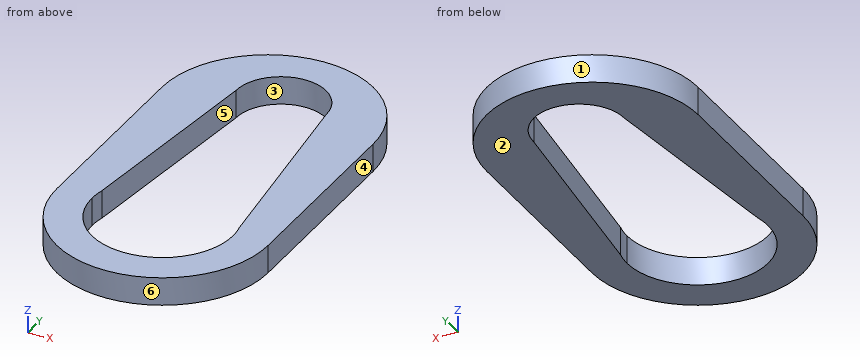
from build123d import *

# Parameters (mm, degrees)
BOSS_EXTRUDE1_DEPTH = 2


with BuildPart() as part:
    # Sketch1 → Boss-Extrude1 (new body)
    with BuildSketch(Plane.XY):
        with BuildLine():
            Line((73.085447554, 74.077647485), (73.085447554, 59.931475915))
            ThreePointArc((73.085447554, 59.931475915), (80.585447554, 52.431475915), (88.085447554, 59.931475915))
            Line((88.085447554, 59.931475915), (88.085447554, 74.077647485))
            ThreePointArc((88.085447554, 74.077647485), (80.585447554, 81.577647485), (73.085447554, 74.077647485))
        make_face()
        with BuildLine():
            Line((75.711262835, 61.046071504), (77.385447554, 75.877647485))
            ThreePointArc((77.385447554, 75.877647485), (80.585447554, 79.077647485), (83.785447554, 75.877647485))
            Line((83.785447554, 75.877647485), (85.459632273, 61.046071504))
            ThreePointArc((85.459632273, 61.046071504), (85.553894172, 60.492312971), (85.585447554, 59.931475915))
            ThreePointArc((85.585447554, 59.931475915), (80.585447554, 54.931475915), (75.585447554, 59.931475915))
            ThreePointArc((75.585447554, 59.931475915), (75.617000936, 60.492312971), (75.711262835, 61.046071504))
        make_face(mode=Mode.SUBTRACT)
    extrude(amount=BOSS_EXTRUDE1_DEPTH)


solid = part.part
Work out the finished part from the listing and answer in its coordinate system (mm). Face numbers are marked on the shaded views. A direction names the side the tool comes from. Round coordinates to 2 decimals unless told otherwise and drop trailing zeros. Write each loop counter-clockwise with the first axis right and the second up, starting at its lowest first coordinate (ties: lowest second). Pieces come first, ordered by that corner, then holes. Notation, with made-up numbers: (-11.75, 52.25) -> (8.25, 52.25) arc R14 ccw to (8.25, 76.25) -> close; hole circle Ø3 at (68.5, -11.5). An arc over 180 degrees is marked (long way). Write each question's results on one line, items separated by ' | '.
Item 1: Which of the six approach directions +Z, -Z, +X, -X, +Y, -Y give full straight-line access (tool end or side, diameter ignored) to the marked faces 5 and 6?
Result set:
face 5: +Z, -Z | face 6: +Z, -Z, -Y
Item 2: A cutting plane is placed at A-A, the plane z = 1.3. Determine the outline of the cut face in (x, y).
Result set:
outline: (73.09, 59.93) arc R7.5 ccw to (88.09, 59.93) -> (88.09, 74.08) arc R7.5 ccw to (73.09, 74.08) -> close; hole (75.71, 61.05) arc R5 ccw (long way) to (85.46, 61.05) -> (83.79, 75.88) arc R3.2 ccw to (77.39, 75.88) -> close
Item 3: A cutting plane is placed at C-C, the plane x = 78. Determine the outline of the cut face in (y, z), plus the area to 3 significant figures.
Result set:
outline: (52.89, 0) -> (55.65, 0) -> (55.65, 2) -> (52.89, 2) -> close; (77.76, 0) -> (81.12, 0) -> (81.12, 2) -> (77.76, 2) -> close | area: 12.2 mm^2
Item 4: Find the intervals of material crossed by line 1 along X through (y, z) = (74.25, 1.75); line 2 along X through (y, z) = (60.25, 1.5); line 3 along Y through (x, z) = (80.5, 0.25), in increasing order. Write a range as [from, to].
Result set:
line 1: [73.09, 77.2], [83.97, 88.08] | line 2: [73.09, 75.6], [85.58, 88.09] | line 3: [52.43, 54.93], [79.08, 81.58]
Item 5: The mould has two halves that part along X. Classify the marked faces 1, 2, 3 and 4: +X half, -X half, draft (parallel to the pull), parting line (faces both ways), or undercut.
Result set:
face 1: parting line | face 2: draft | face 3: undercut | face 4: +X half
Item 6: A cutting plane is placed at D-D, the plane x = 86. Determine the outline of the cut face in (y, z).
Result set:
outline: (54.74, 0) -> (79.27, 0) -> (79.27, 2) -> (54.74, 2) -> close
Item 7: A cutting plane is placed at B-B, the plane y = 68.5. Determine the outline of the cut face in (x, z).
Result set:
outline: (73.09, 0) -> (76.55, 0) -> (76.55, 2) -> (73.09, 2) -> close; (84.62, 0) -> (88.09, 0) -> (88.09, 2) -> (84.62, 2) -> close
